from build123d import *

# Parameters (mm, degrees)
SKETCH2_W           = 26.5
SKETCH2_H           = 16
BOSS_EXTRUDE1_DEPTH = 1.8
SKETCH3_W           = 7
SKETCH3_H           = 16
BOSS_EXTRUDE2_DEPTH = 4.6
SKETCH4_W           = 2
SKETCH4_H           = 2.7
BOSS_EXTRUDE3_DEPTH = 1
SKETCH5_R           = 0.8
SKETCH5_R_2         = 1.2
CUT_EXTRUDE1_DEPTH  = 2.8


with BuildPart() as part:
    # Sketch2 → Boss-Extrude1 (new body)
    with BuildSketch(Plane.XY):
        with Locations((13.25, 8)):
            Rectangle(SKETCH2_W, SKETCH2_H)
    extrude(amount=BOSS_EXTRUDE1_DEPTH)

    # Sketch3 → Boss-Extrude2 (add)
    with BuildSketch(Plane.XY.offset(1.8)):
        with Locations((3.5, 8)):
            Rectangle(SKETCH3_W, SKETCH3_H)
    extrude(amount=BOSS_EXTRUDE2_DEPTH)

    # Sketch4 → Boss-Extrude3 (add)
    with BuildSketch(Plane.XY.offset(1.8)):
        with Locations((18.5, 8)):
            Rectangle(SKETCH4_W, SKETCH4_H)
    extrude(amount=BOSS_EXTRUDE3_DEPTH)

    # Sketch5 → Cut-Extrude1 (cut, through all)
    with BuildSketch(Plane.XY.offset(1.8)):
        with Locations((24.7, 13.25)):
            Circle(SKETCH5_R)
        with Locations((12.7, 2.75)):
            Circle(SKETCH5_R)
        with Locations((24.7, 2.75)):
            Circle(SKETCH5_R_2)
        with Locations((12.7, 13.25)):
            Circle(SKETCH5_R_2)
    extrude(amount=-CUT_EXTRUDE1_DEPTH, mode=Mode.SUBTRACT)


solid = part.part
Part model, mm, in its own coordinate system. A direction names the side the tool comes from. Round coordinates to 2 decimals unless told otherwise and drop trailing zeros. Order: outer loops, then holes, each group sorted by start corner. A loop starts at its lowest first (then second) coordinate and runs counter-clockwise, first axis right, second up. Notation, with made-up numbers: (-26.75, 80) -> (4.25, 80) arc R22 cw to (4.25, 97) -> close; hole circle Ø1 at (-22.5, 42). An arc over 180 degrees is marked (long way). Put each result on its own line as item: value.
Q1. Band-saw the part on C-C (x = 12.7). Give the cut face in (y, z), and give its area (3 significant figures).
From the geometry:
outline: (0, 0) -> (1.95, 0) -> (1.95, 1.8) -> (0, 1.8) -> close; (3.55, 0) -> (12.05, 0) -> (12.05, 1.8) -> (3.55, 1.8) -> close; (14.45, 0) -> (16, 0) -> (16, 1.8) -> (14.45, 1.8) -> close
area: 21.6 mm2
Q2. Wall check: line 1 (Y direction, x = 24.7, z = 0.6); line 2 (Y direction, x = 12.7, z = 0.5); line 3 (X direction, y = 11, z = 5.75). Give the ranges that are in metal, low to high. Write a range as [from, to].
From the geometry:
line 1: y = [0, 1.55], [3.95, 12.45], [14.05, 16]
line 2: y = [0, 1.95], [3.55, 12.05], [14.45, 16]
line 3: x = [0, 7]
Q3. Pull direction Y, two halves, no side cores. Call faces 1 (the face through (18, 9.35, 2)), 2 (the face through (26.5, 8, 1)), 3 (the face through (13.439, 2.444, 0.913)): pulls with the +Y half, pulls with the -Y half, needs draft (parallel to the pull), parting line crosses it, or undercut.
From the geometry:
face 1: pulls with the +Y half
face 2: needs draft
face 3: undercut
Q4. Pin check, flat tips, straight feed: pin 1 Ø1.5 at (x, z) = (12.5, 3) entering from +Y; pin 2 Ø1 at (x, y) = (18.5, 7.5) entering from +Z; pin 3 Ø1.8 at (x, y) = (24.7, 13.25) entering from +Z. Stop position of each tip, or through.
From the geometry:
pin 1: passes through
pin 2: stops at z = 2.8
pin 3: stops at z = 1.8
Q5. Band-saw the part on D-D (x = 18.75). Give the cut face in (y, z), and give its area (3 significant figures).
From the geometry:
outline: (0, 0) -> (16, 0) -> (16, 1.8) -> (9.35, 1.8) -> (9.35, 2.8) -> (6.65, 2.8) -> (6.65, 1.8) -> (0, 1.8) -> close
area: 31.5 mm2
Q6. Band-saw the part on A-A (y = 2.75). Give the cut face in (x, z).
From the geometry:
outline: (0, 0) -> (11.9, 0) -> (11.9, 1.8) -> (7, 1.8) -> (7, 6.4) -> (0, 6.4) -> close; (13.5, 0) -> (23.5, 0) -> (23.5, 1.8) -> (13.5, 1.8) -> close; (25.9, 0) -> (26.5, 0) -> (26.5, 1.8) -> (25.9, 1.8) -> close
Q7. Band-saw the part on B-B (z = 1.5). Give the cut face in (x, y), and give its area (3 significant figures).
From the geometry:
outline: (0, 0) -> (26.5, 0) -> (26.5, 16) -> (0, 16) -> close; hole circle Ø2.4 at (12.7, 13.25); hole circle Ø1.6 at (12.7, 2.75); hole circle Ø2.4 at (24.7, 2.75); hole circle Ø1.6 at (24.7, 13.25)
area: 411 mm2
Q8. Tool access for faces 4 (the face through (18, 6.65, 2)), 5 (the face through (19.5, 8, 2)), 6 (the face through (17.5, 8, 2)): list every direction of +Z, -Z, +X, -X, +Y, -Y with a clear straight run to the whole face (end or side of a thin tool).
From the geometry:
face 4: +Z, +X, -Y
face 5: +Z, +X, +Y, -Y
face 6: +Z, +Y, -Y
